For this review, take the finished solid that the model builds, in its own axes (mm). A direction names the side the tool comes from. Round coordinates to 2 decimals unless told otherwise and drop trailing zeros. Write each loop counter-clockwise with the first axis right and the second up, starting at its lowest first coordinate (ties: lowest second). Pieces come first, ordered by that corner, then holes. Notation, with made-up numbers: (9, 39.5) -> (28, 39.5) arc R14 cw to (28, 48.5) -> close; hole circle Ø4 at (-3.75, -9.75). An arc over 180 degrees is marked (long way). Answer in a Markdown table with one row per item.
from build123d import *

# Parameters (mm, degrees)
F0_W     = 914.4
F0_H     = 19.05
F1_DEPTH = 304.8
F2_W     = 76.2
F2_H     = 76.2
F3_DEPTH = 19.05
F4_W     = 304.8
F4_H     = 19.05
F5_DEPTH = 304.8
F6_W     = 304.8
F6_H     = 19.05
F7_DEPTH = 304.8
F8_W     = 304.8
F8_H     = 19.05
F9_DEPTH = 19.05


with BuildPart() as f1:
    # F0 (on Top) → F1 (new body)
    with BuildSketch(Plane.XY):
        Rectangle(F0_W, F0_H)
    extrude(amount=F1_DEPTH)

    # F2 (on face) → F3 (cut)
    with BuildSketch(Plane.XZ.offset(9.525)):
        with Locations((0, 266.7)):
            Rectangle(F2_W, F2_H)
    extrude(amount=-F3_DEPTH, mode=Mode.SUBTRACT)

    # F4 (on face) → F5 (join)
    with BuildSketch(Plane.XZ.offset(9.525)):
        with Locations((-304.8, 10.287)):
            Rectangle(F4_W, F4_H)
    extrude(amount=F5_DEPTH)

    # F6 (on face) → F7 (join)
    with BuildSketch(Plane.XZ.offset(9.525)):
        with Locations((304.8, 10.287)):
            Rectangle(F6_W, F6_H)
    extrude(amount=F7_DEPTH)

    # F8 (on face) → F9 (join)
    with BuildSketch(Plane.XZ.offset(314.325)):
        Polygon((-152.4, 0.762), (-457.2, 0.762), (-457.2, 0), (457.2, 0), (457.2, 304.8), (-457.2, 304.8), (-457.2, 19.812), (-152.4, 19.812), align=None)
        with Locations((-304.8, 10.287)):
            Rectangle(F8_W, F8_H)
    extrude(amount=F9_DEPTH)


solid = f1.part
1) For line 1 (Y direction, x = 107, z = 50) (3 decimals); line 2 (X direction, y = -220, z = 16); line 3 (Z direction, x = 396, y = -215), list the stretches that pass through material, from the lowest coordinate up. Write a range as [from, to].
Solved:
| item | result |
|---|---|
| line 1 | [-333.375, -314.325], [-9.525, 9.525] |
| line 2 | [-457.2, -152.4], [152.4, 457.2] |
| line 3 | [0.76, 19.81] |
2) Consider section C-C on z = 237. State the section outline as (x, y) points (3 decimals).
Solved:
| item | result |
|---|---|
| outline | (-457.2, -333.375) -> (457.2, -333.375) -> (457.2, -314.325) -> (-457.2, -314.325) -> close; (-457.2, -9.525) -> (-38.1, -9.525) -> (-38.1, 9.525) -> (-457.2, 9.525) -> close; (38.1, -9.525) -> (457.2, -9.525) -> (457.2, 9.525) -> (38.1, 9.525) -> close |
3) Clearance check with flat-ended pins moving along their axes: pin 1 Ø2 at (x, y) = (-153.5, -70.5) entering from +Z; pin 2 Ø5.5 at (x, y) = (-6.5, 0.5) entering from +Z. State where each tip first meets the part, or that it passes through.
Solved:
| item | result |
|---|---|
| pin 1 | z = 19.81 |
| pin 2 | z = 228.6 |
4) Consider section A-A on y = -259. State the section outline as (x, z) points, then the cut area to 3 significant figures.
Solved:
| item | result |
|---|---|
| outline | (-457.2, 0.76) -> (-152.4, 0.76) -> (-152.4, 19.81) -> (-457.2, 19.81) -> close; (152.4, 0.76) -> (457.2, 0.76) -> (457.2, 19.81) -> (152.4, 19.81) -> close |
| area | 11,600 mm² |
5) For faces 5 (the flat face through (303, -160, 19.812)), 6 (the flat face through (-307, -160, 0.762)), 7 (the flat face through (152.4, -160, 10)), list the 3-axis set-ups (+Z, -Z, +X, -X, +Y, -Y) from which the entire face can be reached by the end or side of a thin tool; tool diameter is ignored.
Solved:
| item | result |
|---|---|
| face 5 | +Z, +X, -X |
| face 6 | -Z, +X, -X |
| face 7 | +Z, -Z |
6) Consider section B-B on z = 132. State the section outline as (x, y) points (3 decimals).
Solved:
| item | result |
|---|---|
| outline | (-457.2, -333.375) -> (457.2, -333.375) -> (457.2, -314.325) -> (-457.2, -314.325) -> close; (-457.2, -9.525) -> (457.2, -9.525) -> (457.2, 9.525) -> (-457.2, 9.525) -> close |
7) Mouldability with a two-part tool opening along X and no side actions: class faces 1 (the flat face through (38.1, 0, 266)), 2 (the flat face through (-6, 9.525, 150)), 3 (the flat face through (-38.1, 0, 266)), 4 (the flat face through (457.2, -148, 16)) as pulls with the +X half, pulls with the -X half, needs draft (parallel to the pull), parting line crosses it, or undercut.
Solved:
| item | result |
|---|---|
| face 1 | undercut |
| face 2 | needs draft |
| face 3 | undercut |
| face 4 | pulls with the +X half |
8) Consider section D-D on x = 197. State the section outline as (y, z) points (3 decimals).
Solved:
| item | result |
|---|---|
| outline | (-333.375, 0) -> (-314.325, 0) -> (-314.325, 0.762) -> (-9.525, 0.762) -> (-9.525, 0) -> (9.525, 0) -> (9.525, 304.8) -> (-9.525, 304.8) -> (-9.525, 19.812) -> (-314.325, 19.812) -> (-314.325, 304.8) -> (-333.375, 304.8) -> close |
